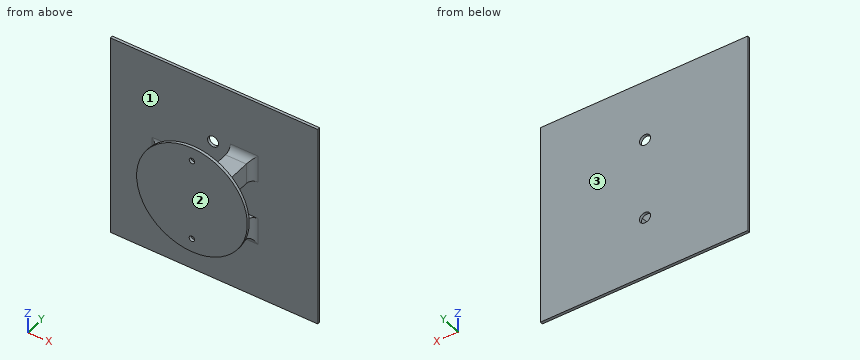
```python
from build123d import *

# Parameters (mm, degrees)
SKETCH1_R                 = 40
BOSS_EXTRUDE1_DEPTH       = 2
F_4_0MM_DOWEL_HOLE1_D     = 4
F_4_0MM_DOWEL_HOLE1_DEPTH = 15
F_4_0MM_DOWEL_HOLE1_TIP   = 1.201721238
SKETCH9_W                 = 15
SKETCH9_H                 = 15
BOSS_EXTRUDE19_DEPTH      = 20
SKETCH10_W                = 150
SKETCH10_H                = 150
BOSS_EXTRUDE20_DEPTH      = 2
SKETCH11_R                = 4
CUT_EXTRUDE1_DEPTH        = 2
FILLET2_R                 = 5


with BuildPart() as part:
    # Sketch1 → Boss-Extrude1 (new body)
    with BuildSketch(Plane(origin=(0, 0, 0), x_dir=(1, 0, 0), z_dir=(0, 1, 0))):
        with Locations(Location((0, 0, 0), (0, 0, 270))):
            Circle(SKETCH1_R)
    extrude(amount=BOSS_EXTRUDE1_DEPTH)

    # Ø4.0mm Dowel Hole1
    with Locations(Plane(origin=(0, 2, 0), x_dir=(1, 0, 0), z_dir=(0, 1, 0))):
        with Locations((0, 30), (0, -30)):
            Hole(F_4_0MM_DOWEL_HOLE1_D / 2, depth=F_4_0MM_DOWEL_HOLE1_DEPTH)
            with Locations((0, 0, -(F_4_0MM_DOWEL_HOLE1_DEPTH + F_4_0MM_DOWEL_HOLE1_TIP / 2))):  # 118° drill point
                Cone(0, F_4_0MM_DOWEL_HOLE1_D / 2, F_4_0MM_DOWEL_HOLE1_TIP, mode=Mode.SUBTRACT)

    # Sketch9 → Boss-Extrude19 (add)
    with BuildSketch(Plane(origin=(0, 2, 0), x_dir=(1, 0, 0), z_dir=(0, 1, 0))):
        with Locations((-31.790584114, 0)):
            Rectangle(SKETCH9_W, SKETCH9_H)
        with Locations((20, -21.547375097)):
            Rectangle(SKETCH9_W, SKETCH9_H)
        with Locations((20, 21.547375097)):
            Rectangle(SKETCH9_W, SKETCH9_H)
    extrude(amount=BOSS_EXTRUDE19_DEPTH)

    # Sketch10 → Boss-Extrude20 (add)
    with BuildSketch(Plane(origin=(0, 22, 0), x_dir=(1, 0, 0), z_dir=(0, 1, 0))):
        with Locations((0.709415886, -0.002124903)):
            Rectangle(SKETCH10_W, SKETCH10_H)
    extrude(amount=BOSS_EXTRUDE20_DEPTH)

    # Sketch11 → Cut-Extrude1 (cut)
    with BuildSketch(Plane.XZ.offset(-22)):
        with Locations(Location((0, 30, 0), (0, 0, 270))):
            Circle(SKETCH11_R)
        with Locations(Location((0, -30, 0), (0, 0, 270))):
            Circle(SKETCH11_R)
    extrude(amount=-CUT_EXTRUDE1_DEPTH, mode=Mode.SUBTRACT)

    # Fillet2
    fillet2_edges = [part.edges().sort_by_distance(p)[0] for p in [
        (-39.290584114, 22, 0),
        (-31.790584114, 22, 7.5),
        (-31.790584114, 22, -7.5),
        (27.5, 22, 21.547375097),
        (20, 22, 29.047375097),
        (20, 22, -29.047375097),
        (27.5, 22, -21.547375097),
    ]]
    fillet(fillet2_edges, radius=FILLET2_R)


solid = part.part
```
Input: part model. Units: mm. Frame: model coordinates. Face numbers are marked on the shaded views. Give positions to 0.01 mm unless a question says otherwise; leave off trailing zeros. Order: outer loops, then holes, each group sorted by start corner. A loop starts at its lowest first (then second) coordinate and runs counter-clockwise, first axis right, second up.
1. Cut plane A-A (x = 0). Return loops of the section in (y, z).
Computed:
outline: (0, -40) - (2, -40) - (2, -32) - (0, -32) - close; (0, -28) - (2, -28) - (2, 28) - (0, 28) - close; (0, 32) - (2, 32) - (2, 40) - (0, 40) - close; (22, -75) - (24, -75) - (24, -34) - (22, -34) - close; (22, -26) - (24, -26) - (24, 26) - (22, 26) - close; (22, 34) - (24, 34) - (24, 75) - (22, 75) - close
2. Draft query along Y for the marked faces 1, 2 and 3. Return one class per face: released by +Y, released by -Y, zero draft, split by the parting line, or undercut.
Computed:
face 1: undercut
face 2: released by -Y
face 3: released by +Y
3. Pin query (flat end, axial travel): pin 1 Ø7.5 at (y, z) = (11.5, 21) entering from +X; pin 2 Ø6.5 at (x, z) = (0, -30) entering from +Y; pin 3 Ø4.5 at (x, y) = (19.5, 11.5) entering from +Z. Return the tip coordinate at first contact, or that it passes through.
Computed:
pin 1: stops at x = 27.5
pin 2: stops at y = 2
pin 3: stops at z = 29.05
4. Cut plane B-B (y = 4.25). Return loops of the section in (x, z).
Computed:
outline: (-39.29, -7.5) - (-24.29, -7.5) - (-24.29, 7.5) - (-39.29, 7.5) - close; (12.5, -29.05) - (27.5, -29.05) - (27.5, -14.05) - (12.5, -14.05) - close; (12.5, 14.05) - (27.5, 14.05) - (27.5, 29.05) - (12.5, 29.05) - close
5. Cut plane C-C (z = 0). Return loops of the section in (x, y).
Computed:
outline: (-74.29, 22) - (-44.29, 22) arc R5 cw to (-39.29, 17) - (-39.29, 2) - (-40, 2) - (-40, 0) - (40, 0) - (40, 2) - (-24.29, 2) - (-24.29, 22) - (75.71, 22) - (75.71, 24) - (-74.29, 24) - close
6. Cut plane D-D (y = 20). Return loops of the section in (x, z).
Computed:
outline: (-40.29, -8.5) - (-24.29, -8.5) - (-24.29, 8.5) - (-40.29, 8.5) - close; (12.5, -30.05) - (28.5, -30.05) - (28.5, -14.05) - (12.5, -14.05) - close; (12.5, 14.05) - (28.5, 14.05) - (28.5, 30.05) - (12.5, 30.05) - close
7. Line query: probe 1 along Z at (x, y) = (0, 1.4); probe 2 along X at (y, z) = (23.55, 30); probe 3 along Y at (x, z) = (55.5, -9.5). Output: solid intervals per line, ascending.
Computed:
probe 1: z = -40 to -32, -28 to 28, 32 to 40
probe 2: x = -74.29 to -4, 4 to 75.71
probe 3: y = 22 to 24
